The figure shows three views and two pictorial views of one solid part (mm, origin at its lowest corner). Answer the questions. A direction names the side the tool comes from. Round coordinates to 2 decimals unless told otherwise and drop trailing zeros. Order: outer loops, then holes, each group sorted by start corner. A loop starts at its lowest first (then second) coordinate and runs counter-clockwise, first axis right, second up. Notation, with made-up numbers: (79, -33.5) -> (97, -33.5) arc R19 cw to (97, -10.5) -> close; hole circle Ø1 at (43, -27). An arc over 180 degrees is marked (long way). Answer as a JSON object with one key per item and string values. Group by question number.
Item 1: For the marked faces 4, 5 and 6, determine the directions among +Z, -Z, +X, -X, +Y, -Y from which every point of the face is accessible in a straight line to the end or side of a thin tool.
Item 2: Section A-A, the plane y = 3.75 is taken. Write down the section's boundary in (x, z).
Item 3: Section B-B, the plane x = 17.75 is taken. Write down the section's boundary in (y, z), plus the area to 3 significant figures.
Item 4: The mould has two halves that part along Y. Classify the marked faces 1, 2 and 3: pulls with the +Y half, pulls with the -Y half, needs draft (parallel to the pull), parting line crosses it, or undercut.
Item 5: Section C-C, the plane y = 9.75 is taken. Write down the section's boundary in (x, z), plus the area to 3 significant figures.
Item 6: Consider probe 1 along Y at (x, z) = (3, 5.5); probe 2 along X at (y, z) = (2, 1.5); probe 3 along Z at (x, y) = (18.5, 2.75). Determine where each line is inside the solid, lowest interval first. Write a range as from..to.
Item 7: Given P1, Ø5, axis at x = 16.5, y = 6.5, coming from the -Z side; P2, Ø5, axis at x = 5.5, y = 4.5, coming from the -Z side; P3, Ø4, axis at x = 16.5, y = 6.5, coming from the +Z side, each flat-ended and moving along its own axis, determine where each tip first touches the part or whether it passes through.
Item 8: Section D-D, the plane z = 6.25 is taken. Write down the section's boundary in (x, y) (1 decimal), plus the area to 3 significant figures.
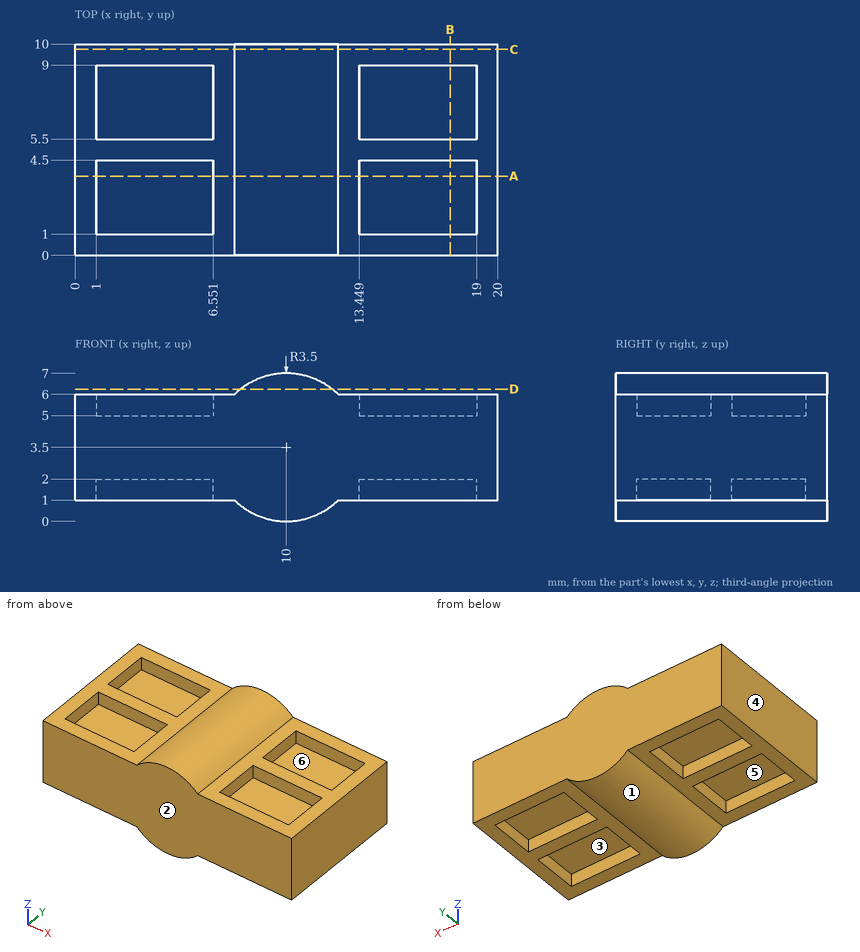
Values found:
{
 "1": {"face 4": "+Z, -Z, -X, +Y, -Y", "face 5": "-Z", "face 6": "+Z"},
 "2": {"outline": "(0, 1) -> (1, 1) -> (1, 2) -> (6.55, 2) -> (6.55, 1) -> (7.55, 1) arc R3.5 ccw to (12.45, 1) -> (13.45, 1) -> (13.45, 2) -> (19, 2) -> (19, 1) -> (20, 1) -> (20, 6) -> (19, 6) -> (19, 5) -> (13.45, 5) -> (13.45, 6) -> (12.45, 6) arc R3.5 ccw to (7.55, 6) -> (6.55, 6) -> (6.55, 5) -> (1, 5) -> (1, 6) -> (0, 6) -> close"},
 "3": {"outline": "(0, 1) -> (1, 1) -> (1, 2) -> (4.5, 2) -> (4.5, 1) -> (5.5, 1) -> (5.5, 2) -> (9, 2) -> (9, 1) -> (10, 1) -> (10, 6) -> (9, 6) -> (9, 5) -> (5.5, 5) -> (5.5, 6) -> (4.5, 6) -> (4.5, 5) -> (1, 5) -> (1, 6) -> (0, 6) -> close", "area": "36.0 mm2"},
 "4": {"face 1": "needs draft", "face 2": "pulls with the -Y half", "face 3": "undercut"},
 "5": {"outline": "(0, 1) -> (7.55, 1) arc R3.5 ccw to (12.45, 1) -> (20, 1) -> (20, 6) -> (12.45, 6) arc R3.5 ccw to (7.55, 6) -> (0, 6) -> close", "area": "107 mm2"},
 "6": {"probe 1": "0..1, 4.5..5.5, 9..10", "probe 2": "0..1, 6.55..13.45, 19..20", "probe 3": "2..5"},
 "7": {"P1": "z = 1", "P2": "z = 0.63", "P3": "z = 6"},
 "8": {"outline": "(7.8, 0) -> (12.2, 0) -> (12.2, 10) -> (7.8, 10) -> close", "area": "43.3 mm2"}
}
